Could you check a few things on this model? Use its own coordinates, in mm. A direction names the side the tool comes from. Coordinates: 2 decimals unless noted, no trailing zeros. Order: outer loops, then holes, each group sorted by start corner. A loop starts at its lowest first (then second) coordinate and runs counter-clockwise, first axis right, second up. Notation, with made-up numbers: (89, 71) -> (93, 71) arc R27 ccw to (93, 107) -> close; hole circle Ø11 at (54.5, -11.75). An arc over 180 degrees is marked (long way). Return JSON: item names as keys, results as strings. Group by question number.
from build123d import *

# Parameters (mm, degrees)
CROQUIS1_R                                           = 9.525
SALIENTE_EXTRUIR1_DEPTH                              = 63.5
CROQUIS2_W                                           = 19.05
CROQUIS2_H                                           = 20.32
CORTAR_EXTRUIR1_DEPTH                                = 15.748
CORTAR_EXTRUIR2_DEPTH                                = 15.748
TALADRO_ROSCADO_5_16_181_D                           = 6.5278
TALADRO_ROSCADO_5_16_181_DEPTH                       = 22.9235
TALADRO_ROSCADO_5_16_181_TIP                         = 1.961148974
CROQUIS6_W                                           = 19.05
CROQUIS6_H                                           = 20.32
CORTAR_EXTRUIR3_DEPTH                                = 19.05
CORTAR_EXTRUIR4_DEPTH                                = 19.05
REFRENTADO_PARA_TORNILLO_CON_CABEZA_HUEC_D           = 8.2042
REFRENTADO_PARA_TORNILLO_CON_CABEZA_HUEC_DEPTH       = 9.398
REFRENTADO_PARA_TORNILLO_CON_CABEZA_HUEC_CBORE_D     = 12.446
REFRENTADO_PARA_TORNILLO_CON_CABEZA_HUEC_CBORE_DEPTH = 7.9375
REFRENTADO_PARA_TORNILLO_CON_CABEZA_HUEC_TIP         = 2.464790345


with BuildPart() as part:
    # Croquis1 → Saliente-Extruir1 (new body)
    with BuildSketch(Plane(origin=(0, 0, 0), x_dir=(1, 0, 0), z_dir=(0, 1, 0))):
        with Locations(Location((0, 0, 0), (0, 0, 270))):
            Circle(CROQUIS1_R)
    extrude(amount=SALIENTE_EXTRUIR1_DEPTH)

    # Croquis2 → Cortar-Extruir1 (cut)
    with BuildSketch(Plane.XY):
        with Locations((0, 53.34)):
            Rectangle(CROQUIS2_W, CROQUIS2_H)
    extrude(amount=-CORTAR_EXTRUIR1_DEPTH, mode=Mode.SUBTRACT)

    # Croquis3 → Cortar-Extruir2 (cut)
    with BuildSketch(Plane(origin=(0, 0, 0), x_dir=(-1, 0, 0), z_dir=(0, 0, -1))):
        with BuildLine():
            Line((-9.525, 63.5), (-9.525, 53.975))
            ThreePointArc((-9.525, 53.975), (-6.735192091, 60.710192091), (0, 63.5))
            Line((0, 63.5), (-9.525, 63.5))
        make_face()
        with BuildLine():
            Line((9.525, 63.5), (0, 63.5))
            ThreePointArc((0, 63.5), (6.735192091, 60.710192091), (9.525, 53.975))
            Line((9.525, 53.975), (9.525, 63.5))
        make_face()
    extrude(amount=-CORTAR_EXTRUIR2_DEPTH, mode=Mode.SUBTRACT)

    # Taladro roscado 5/16-181
    with Locations(Plane(origin=(0, 0, 0), x_dir=(-1, 0, 0), z_dir=(0, 0, -1))):
        with Locations((0, 53.975)):
            Hole(TALADRO_ROSCADO_5_16_181_D / 2, depth=TALADRO_ROSCADO_5_16_181_DEPTH)
            with Locations((0, 0, -(TALADRO_ROSCADO_5_16_181_DEPTH + TALADRO_ROSCADO_5_16_181_TIP / 2))):  # 118° drill point
                Cone(0, TALADRO_ROSCADO_5_16_181_D / 2, TALADRO_ROSCADO_5_16_181_TIP, mode=Mode.SUBTRACT)

    # Croquis6 → Cortar-Extruir3 (cut)
    with BuildSketch(Plane.XY):
        with Locations((0, 10.16)):
            Rectangle(CROQUIS6_W, CROQUIS6_H)
    extrude(amount=CORTAR_EXTRUIR3_DEPTH, mode=Mode.SUBTRACT)

    # Croquis7 → Cortar-Extruir4 (cut)
    with BuildSketch(Plane.XY):
        with BuildLine():
            ThreePointArc((-3.4e-08, 0), (-6.735192103, 2.789807921), (-9.525, 9.525))
            Line((-9.525, 9.525), (-9.525, 0))
            Line((-9.525, 0), (-3.4e-08, 0))
        make_face()
        with BuildLine():
            ThreePointArc((9.525, 9.525), (6.735192079, 2.789807897), (-3.4e-08, 0))
            Line((-3.4e-08, 0), (9.525, 0))
            Line((9.525, 0), (9.525, 9.525))
        make_face()
    extrude(amount=-CORTAR_EXTRUIR4_DEPTH, mode=Mode.SUBTRACT)

    # Refrentado para tornillo con cabeza hueca de 5/161
    with Locations(Plane(origin=(0, 0, -9.525), x_dir=(-1, 0, 0), z_dir=(0, 0, -1))):
        with Locations((0, 9.525)):
            CounterBoreHole(REFRENTADO_PARA_TORNILLO_CON_CABEZA_HUEC_D / 2, REFRENTADO_PARA_TORNILLO_CON_CABEZA_HUEC_CBORE_D / 2, REFRENTADO_PARA_TORNILLO_CON_CABEZA_HUEC_CBORE_DEPTH, depth=REFRENTADO_PARA_TORNILLO_CON_CABEZA_HUEC_DEPTH)
            with Locations((0, 0, -(REFRENTADO_PARA_TORNILLO_CON_CABEZA_HUEC_DEPTH + REFRENTADO_PARA_TORNILLO_CON_CABEZA_HUEC_TIP / 2))):  # 118° drill point
                Cone(0, REFRENTADO_PARA_TORNILLO_CON_CABEZA_HUEC_D / 2, REFRENTADO_PARA_TORNILLO_CON_CABEZA_HUEC_TIP, mode=Mode.SUBTRACT)


solid = part.part
Q1. I want a section at B-B on z = 7.25. Please give me the cut outline in (x, y) (3 decimals).
Q2. I want a section at D-D on x = -1. State how many separate pieces and enclosed holes the cut face has, and give its area (3 significant figures).
Q3. We'd pull the mould along X, two halves only. Please class faces 5 (the cylindrical face through (8.03, 31.31, 5.12)), 6 (the flat face through (2, 51, 0)), 7 (the flat face through (-1, 5, -1.588)): pulls with the +X half, pulls with the -X half, needs draft (parallel to the pull), parting line crosses it, or undercut.
Q4. I need wall thicknesses on line 1 along Y through (x, z) = (0, -5.5); line 2 along Y through (x, z) = (-5.5, -5.5); line 3 along X through (y, z) = (29, 5.5). Which ranges of each line are inside material? Lowest first, please. Write a range as from..to.
Q5. On a 3-axis mill with a long thin cutter (end or side, diameter ignored), from which of +Z, -Z, +X, -X, +Y, -Y can I reach the whole of each face in a straight line? I mean faces 1 (the flat face through (0, 43.18, -4)), 2 (the cylindrical face through (-3.26, 54.12, 4.83)), 3 (the cylindrical face through (-0.534, 13.592, -0.847)), 4 (the flat face through (0, 20.32, 4)). Say none if no direction works.
Q6. I'm going to push flat-ended pins straight in: pin 1 Ø8 at (y, z) = (42, 5.5) entering from +X; pin 2 Ø4 at (x, y) = (0, 53.975) entering from -Z; pin 3 Ø5 at (x, z) = (2.5, 3) entering from +Y; pin 4 Ø3 at (x, z) = (-1, 7) entering from -Y. Where does each tip first touch, or does it pass through?
Q7. I want a section at A-A on x = 5. Please give me the cut outline in (y, z).
Q8. I want a section at C-C on y = 29.5. Please give me the cut outline in (x, z) (3 decimals).
Response values:
{
 "1": {"outline": "(-6.178, 20.32) -> (6.178, 20.32) -> (6.178, 61.225) arc R9.525 ccw to (-6.178, 61.225) -> close; hole circle Ø6.528 at (0, 53.975)"},
 "2": {"separate pieces": "3", "enclosed holes": "0", "area": "649 mm²"},
 "3": {"face 5": "parting line crosses it", "face 6": "needs draft", "face 7": "undercut"},
 "4": {"line 1": "y = 0..3.3, 15.75..43.18", "line 2": "y = 1.75..6.61, 12.44..43.18", "line 3": "x = -7.78..7.78"},
 "5": {"face 1": "-Z, +X, -X, +Y", "face 2": "+Z, -Z", "face 3": "-Z", "face 4": "+Z, +X, -X, -Y"},
 "6": {"pin 1": "stops at x = 9.41", "pin 2": "passes through", "pin 3": "stops at y = 63.5", "pin 4": "stops at y = 20.32"},
 "7": {"outline": "(1.42, -8.11) -> (5.82, -8.11) -> (5.82, -1.59) -> (13.23, -1.59) -> (13.23, -8.11) -> (43.18, -8.11) -> (43.18, 0) -> (62.08, 0) -> (62.08, 8.11) -> (20.32, 8.11) -> (20.32, 0) -> (1.42, 0) -> close"},
 "8": {"outline": "circle Ø19.05 at (0, 0)"}
}
